Part model, mm, in its own coordinate system. Give positions to 0.01 mm unless a question says otherwise; leave off trailing zeros. Write each loop counter-clockwise with the first axis right and the second up, starting at its lowest first coordinate (ties: lowest second). Pieces come first, ordered by that corner, then holes. Notation, with made-up numbers: M 54,78.5 L 92,78.5 A9 cw 92,94.5 Z; hole C 29.5,88.5 d6. An arc over 180 degrees is marked long. Use CSV: the item, a comma, the result in double quotes. Start each with the question number.
1. Band-saw the part on B-B, the plane y = 123. List the corners of the cut face in (x, z) (3 decimals), then the cut area to 3 significant figures.
2. Drop flat-ended pins along their axis: pin 1 Ø1 at (x, z) = (100, 2) entering from -Y (3 decimals); pin 2 Ø4 at (x, y) = (167, 113) entering from -Z. Give the stop position or say it passes through.
3. Band-saw the part on D-D, the plane z = 2. Count the separate pieces of the cut face and the enclosed holes in it, then the cut area to 3 significant figures.
4. Band-saw the part on A-A, the plane x = 224. List the corners of the cut face in (y, z) (3 decimals).
5. Drill centre lines: line 1 along X through (y, z) = (135.75, 0.85) (3 decimals); line 2 along Y through (x, z) = (246, 2.4) (3 decimals); line 3 along Y through (x, z) = (513.5, 2.3). Where is each one in solid material? Low to high. Write a range as from..to.
6. Band-saw the part on C-C, the plane x = 512.5. List the corners of the cut face in (y, z) (3 decimals).
from build123d import *

# Parameters (mm, degrees)
SKETCH1_R           = 1.5
SKETCH1_W           = 71.428571428
SKETCH1_H           = 3.175
SKETCH1_W_2         = 20
SKETCH1_W_3         = 13.333
SKETCH1_W_4         = 42.3
SKETCH1_H_2         = 44.35
SKETCH1_W_5         = 18.5
BOSS_EXTRUDE1_DEPTH = 3.175


with BuildPart() as part:
    # Sketch1 → Boss-Extrude1 (new body)
    with BuildSketch(Plane.XY):
        Polygon((0, 0), (0, 132.75), (0, 252.75), (328.222222222, 252.75), (363, 252.75), (363, 228.115), (363, 132.75), (357.142857143, 132.75), (357.142857143, 129.575), (428.571428571, 129.575), (428.571428571, 132.75), (550, 132.75), (550, 0), (428.571428571, 0), (428.571428571, 3.175), (357.142857143, 3.175), (357.142857143, 0), (285.714285714, 0), (285.714285714, 3.175), (214.285714286, 3.175), (214.285714286, 0), (142.857142857, 0), (142.857142857, 3.175), (71.428571429, 3.175), (71.428571429, 0), align=None)
        with Locations((56.175, 246.575)):
            Circle(SKETCH1_R, mode=Mode.SUBTRACT)
        with Locations((158.920833333, 135.75)):
            Circle(SKETCH1_R, mode=Mode.SUBTRACT)
        with Locations((158.920833333, 246.575)):
            Circle(SKETCH1_R, mode=Mode.SUBTRACT)
        with Locations((254.079166667, 246.575)):
            Circle(SKETCH1_R, mode=Mode.SUBTRACT)
        with Locations((254.079166667, 135.75)):
            Circle(SKETCH1_R, mode=Mode.SUBTRACT)
        with Locations((356.825, 135.75)):
            Circle(SKETCH1_R, mode=Mode.SUBTRACT)
        with Locations((356.825, 246.575)):
            Circle(SKETCH1_R, mode=Mode.SUBTRACT)
        with Locations((56.175, 135.75)):
            Circle(SKETCH1_R, mode=Mode.SUBTRACT)
        with Locations((107.142857143, 131.1625)):
            Rectangle(SKETCH1_W, SKETCH1_H, mode=Mode.SUBTRACT)
        with Locations((250, 131.1625)):
            Rectangle(SKETCH1_W, SKETCH1_H, mode=Mode.SUBTRACT)
        with Locations((536, 60.0875)):
            Rectangle(SKETCH1_W_2, SKETCH1_H, mode=Mode.SUBTRACT)
        with Locations((536, 72.6625)):
            Rectangle(SKETCH1_W_2, SKETCH1_H, mode=Mode.SUBTRACT)
        with Locations((532.6665, 16.5875)):
            Rectangle(SKETCH1_W_3, SKETCH1_H, mode=Mode.SUBTRACT)
        with Locations((24.95, 112.68)):
            Rectangle(SKETCH1_W_4, SKETCH1_H_2, mode=Mode.SUBTRACT)
        with Locations((32.933020508, 56.5875)):
            Rectangle(SKETCH1_W_5, SKETCH1_H, mode=Mode.SUBTRACT)
        with Locations((35.516520508, 16.5875)):
            Rectangle(SKETCH1_W_3, SKETCH1_H, mode=Mode.SUBTRACT)
        with Locations((35.516520508, 39.7625)):
            Rectangle(SKETCH1_W_3, SKETCH1_H, mode=Mode.SUBTRACT)
        with Locations((532.6665, 39.7625)):
            Rectangle(SKETCH1_W_3, SKETCH1_H, mode=Mode.SUBTRACT)
    extrude(amount=BOSS_EXTRUDE1_DEPTH)


solid = part.part
Output:
1,outline,"M 0,0 L 3.8,0 L 3.8,3.175 L 0,3.175 Z; M 46.1,0 L 550,0 L 550,3.175 L 46.1,3.175 Z"
1,area,"1,610 mm²"
2,pin 1,"stops at y = 3.175"
2,pin 2,"stops at z = 0"
3,separate pieces,"1"
3,enclosed holes,"18"
3,area,"113,000 mm²"
4,outline,"M 3.175,0 L 129.575,0 L 129.575,3.175 L 3.175,3.175 Z; M 132.75,0 L 252.75,0 L 252.75,3.175 L 132.75,3.175 Z"
5,line 1,"x = 0..54.675, 57.675..157.421, 160.421..252.579, 255.579..355.325, 358.325..363"
5,line 2,"y = 3.175..129.575, 132.75..252.75"
5,line 3,"y = 0..132.75"
6,outline,"M 0,0 L 132.75,0 L 132.75,3.175 L 0,3.175 Z"
